The listing builds one solid part. Answer for the finished solid, in the listing's coordinates (mm). A direction names the side the tool comes from. Give positions to 0.01 mm unless a question says otherwise; leave off trailing zeros. Write each loop counter-clockwise with the first axis right and the second up, starting at its lowest first coordinate (ties: lowest second). Pieces come first, ordered by that corner, then holes. Notation, with made-up numbers: (79.5, 32.5) -> (90.5, 32.5) arc R13 ccw to (90.5, 54.5) -> close; hole circle Ø3 at (38.5, 28). An arc over 180 degrees is marked (long way). Put each result on its own line as item: value. Start each with the question number.
1) For faces 1 (the flat face through (55, 132.551, 37)), 2 (the flat face through (-40.961, 50, 35)), determine the directions among +Z, -Z, +X, -X, +Y, -Y from which every point of the face is accessible in a straight line to the end or side of a thin tool.
2) A cutting plane is placed at A-A (z = 39). Write down the section's boundary in (x, y), then the cut area to 4 significant figures.
3) A flat-ended cylindrical pin translates along its axis: pin 1 Ø1.5 at (x, y) = (9.5, 59.5) entering from +Z. Find the tip coordinate at first contact, or state that the pin passes through.
4) For a pull along Y with two mould halves and no side action, classify faces 3 (the flat face through (55, -30.36, 37)), 4 (the flat face through (153.129, 50, 35)), 5 (the flat face through (150.629, 50, 37)), 6 (the flat face through (55, -32.86, 35)) as released by +Y, released by -Y, zero draft, split by the parting line, or undercut.
5) Find the intervals of material crossed by line 1 along X through (y, z) = (125.5, 16); line 2 along Y through (x, z) = (80, 47.5); line 3 along Z through (x, y) = (-17, -20), in increasing order. Write a range as from..to.
6) A cutting plane is placed at C-C (x = -8.5). Write down the section's boundary in (y, z).
7) A cutting plane is placed at B-B (y = 19). Write down the section's boundary in (x, z).
from build123d import *

# Parameters (mm, degrees)
F0_W     = 113.0900681019
F0_H     = 62.9108082503
F1_DEPTH = 71.882
F2_DEPTH = 81
F3_DEPTH = 105
F4_T     = -2.5


with BuildPart() as f1:
    # F0 (on Top) → F1 (new body)
    with BuildSketch(Plane.XY):
        with Locations((15.5839696527, -1.4044689015)):
            Rectangle(F0_W, F0_H)
    extrude(amount=F1_DEPTH)

    # F2 (add): a face of the model
    f2_faces = [f1.faces().sort_by_distance(p)[0] for p in [
        (72.1290037036, -1.4044689015, 35.941),
    ]]
    extrude(f2_faces, amount=F2_DEPTH)

    # F3 (add): a face of the model
    f3_faces = [f1.faces().sort_by_distance(p)[0] for p in [
        (56.0839696527, 30.0509352237, 35.941),
    ]]
    extrude(f3_faces, amount=F3_DEPTH)

    # F4
    f4_openings = [f1.faces().sort_by_distance(p)[0] for p in [
        (56.08397, 51.095531, 71.882),
    ]]
    offset(amount=F4_T, openings=f4_openings)


solid = f1.part
Reply:
1. face 1: +Z
1. face 2: +Z, -Z, -X, +Y, -Y
2. outline: (-40.96, -32.86) -> (153.13, -32.86) -> (153.13, 135.05) -> (-40.96, 135.05) -> close; hole (-38.46, -30.36) -> (150.63, -30.36) -> (150.63, 132.55) -> (-38.46, 132.55) -> close
2. area: 1,785 mm2
3. pin 1: stops at z = 2.5
4. face 3: undercut
4. face 4: zero draft
4. face 5: undercut
4. face 6: released by -Y
5. line 1: x = -40.96..-38.46, 150.63..153.13
5. line 2: y = -32.86..-30.36, 132.55..135.05
5. line 3: z = 0..2.5
6. outline: (-32.86, 0) -> (135.05, 0) -> (135.05, 71.88) -> (132.55, 71.88) -> (132.55, 2.5) -> (-30.36, 2.5) -> (-30.36, 71.88) -> (-32.86, 71.88) -> close
7. outline: (-40.96, 0) -> (153.13, 0) -> (153.13, 71.88) -> (150.63, 71.88) -> (150.63, 2.5) -> (-38.46, 2.5) -> (-38.46, 71.88) -> (-40.96, 71.88) -> close
